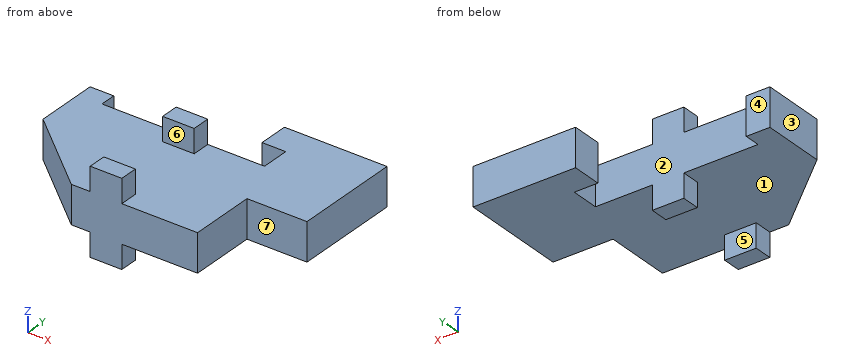
```python
from build123d import *

# Parameters (mm, degrees)
F1_DEPTH = 1.2
F2_W     = 2
F2_H     = 1.15
F3_DEPTH = 1.5


# Not quite as in the source:
# - a pattern or mirror of a feature is missing from the dataset's text; its kind, count and spacing are read off the source's solid


with BuildPart() as f1:
    # F0 (on Top) → F1 (new body, symmetric)
    with BuildSketch(Plane.XY):
        Polygon((0, 4.2), (0, 11), (-6.5, 11), (-6.5, 9.1), (-5, 9.1), (-5, 7.3), (-15.3, 7.3), (-15.3, 8.3), (-16.8, 8.3), (-16.8, 4.3), (-11.8, 0), (-3.8, 0), (-3.8, 4.2), align=None)
    extrude(amount=F1_DEPTH, both=True)

    # F2 (on face) → F3 (join)
    with BuildSketch(Plane.XY.offset(1.2)):
        with Locations((-9.6, 0.575)):
            Rectangle(F2_W, F2_H)
        with Locations((-9.6, 6.725)):
            Rectangle(F2_W, F2_H)
    f3 = extrude(amount=F3_DEPTH)

    # F3_copies: F3 across plane
    add(f3.mirror(Plane(origin=(0, 0, 0), x_dir=(-1, 0, 0), z_dir=(0, 0, -1))))


solid = f1.part
```
Can you work these out from the model? Positions are in its coordinate system, mm. Face numbers are marked on the shaded views. A direction names the side the tool comes from. Give positions to 0.01 mm unless a question says otherwise; leave off trailing zeros. Order: outer loops, then holes, each group sorted by start corner. A loop starts at its lowest first (then second) coordinate and runs counter-clockwise, first axis right, second up. Notation, with made-up numbers: (31.5, 84.25) - (44.5, 84.25) arc R15 ccw to (44.5, 103.25) - close; hole circle Ø11 at (78, -13). An arc over 180 degrees is marked (long way). Use a Markdown table: item, result. Add a question column.
Q1. If we section it at C-C on y = 6.5: Write out the boundary of the cut face in (x, z), plus the area to 3 significant figures.
Q2. I'm going to push flat-ended pins straight in: pin 1 (0.9 mm diameter, centred on y = 0.5, z = 1.5, fed in from -X); pin 2 (1.3 mm diameter, centred on y = 7, z = -2, fed in from +X); pin 3 (2 mm diameter, centred on y = 10, z = 0, fed in from -X). Where does each tip first touch, or does it pass through?
Q3. On a 3-axis mill with a long thin cutter (end or side, diameter ignored), from which of +Z, -Z, +X, -X, +Y, -Y can I reach the whole of each face in a straight line? I mean the marked faces 4, 5, 6 and 7. Say none if no direction works.
Q4. If we section it at D-D on z = 0.5: Write out the boundary of the cut face in (x, y).
Q5. If we mould it in two halves opening along X, with no side actions, what happens to the marked faces 1, 2 and 3? For each: released by +X, released by -X, zero draft, split by the parting line, or undercut.
Q6. If we section it at A-A on y = 7.75: Write out the boundary of the cut face in (x, z).
Q7. If we section it at B-B on z = 2.35: Write out the boundary of the cut face in (x, y).
Q8. Please list where these lines run through material, in increasing order: line 1 along Y through (x, z) = (-5.25, -0.75); line 2 along Z through (x, y) = (-2.5, 6.5); line 3 along X through (y, z) = (9.5, 0.1).
Answers follow:
| question | item | result |
|---|---|---|
| 1 | outline | (-16.8, -1.2) - (-10.6, -1.2) - (-10.6, -2.7) - (-8.6, -2.7) - (-8.6, -1.2) - (0, -1.2) - (0, 1.2) - (-8.6, 1.2) - (-8.6, 2.7) - (-10.6, 2.7) - (-10.6, 1.2) - (-16.8, 1.2) - close |
| 1 | area | 46.3 mm^2 |
| 2 | pin 1 | stops at x = -12.77 |
| 2 | pin 2 | stops at x = -8.6 |
| 2 | pin 3 | stops at x = -6.5 |
| 3 | face 4 | +Z, -Z, -X, +Y |
| 3 | face 5 | -Z, +X, -X |
| 3 | face 6 | +Z, +X, -X |
| 3 | face 7 | +Z, -Z, +X, -Y |
| 4 | outline | (-16.8, 4.3) - (-11.8, 0) - (-3.8, 0) - (-3.8, 4.2) - (0, 4.2) - (0, 11) - (-6.5, 11) - (-6.5, 9.1) - (-5, 9.1) - (-5, 7.3) - (-15.3, 7.3) - (-15.3, 8.3) - (-16.8, 8.3) - close |
| 5 | face 1 | zero draft |
| 5 | face 2 | undercut |
| 5 | face 3 | released by -X |
| 6 | outline | (-16.8, -1.2) - (-15.3, -1.2) - (-15.3, 1.2) - (-16.8, 1.2) - close; (-5, -1.2) - (0, -1.2) - (0, 1.2) - (-5, 1.2) - close |
| 7 | outline | (-10.6, 0) - (-8.6, 0) - (-8.6, 1.15) - (-10.6, 1.15) - close; (-10.6, 6.15) - (-8.6, 6.15) - (-8.6, 7.3) - (-10.6, 7.3) - close |
| 8 | line 1 | y = 0 to 7.3, 9.1 to 11 |
| 8 | line 2 | z = -1.2 to 1.2 |
| 8 | line 3 | x = -6.5 to 0 |
